For this review, use the dimensioned drawing (mm, ordinates from the lowest corner) and the shaded views. A direction names the side the tool comes from. Round coordinates to 2 decimals unless told otherwise and drop trailing zeros. Write each loop counter-clockwise with the first axis right and the second up, starting at its lowest first coordinate (ties: lowest second). Pieces come first, ordered by that corner, then holes. Notation, with made-up numbers: M -34,78.5 L 12,78.5 A29 ccw 12,100.5 Z; hole C 78.5,31.5 d8. An arc over 180 degrees is marked long. One line per question, with ' | ' between items. Start each with the question number.
Item 1: Add section D-D, the plane y = 50. State the section outline as (x, z) points.
Item 2: Add section A-A, the plane z = 9.5. State the section outline as (x, y) points, and give its area (3 significant figures).
Item 3: Machinability: for the marked faces 4 and 5, which of the approach directions +Z, -Z, +X, -X, +Y, -Y give a long, thin tool a straight path to every point of the face, cutting with its end or side? Answer none if there is none.
Item 4: Add section C-C, the plane x = 3. State the section outline as (y, z) points.
Item 5: For L1, parallel to X at y = 58, z = 16.75; L2, parallel to Z at x = 27, y = 31, list the stretches that pass through material, from the lowest coordinate up.
Item 6: Draft analysis for pull direction Y (two halves, no side actions). For the marked faces 1, 2 and 3, state which applies: released by +Y, released by -Y, zero draft, split by the parting line, or undercut.
Item 7: Add section B-B, the plane y = 65. State the section outline as (x, z) points, and give its area (3 significant figures).
Item 8: Insertion check: pin 1 Ø1 at (y, z) = (0.5, 9) entering from -X; pin 2 Ø1 at (x, y) = (7, 32) entering from +Z; pin 3 Ø5 at (x, z) = (31.5, 6.5) entering from +Y; pin 4 Ø5 at (y, z) = (32.5, 16.5) entering from +X. Each pin has a flat end and moves straight along its axis. Give the tip position at first contact, or say it passes through.
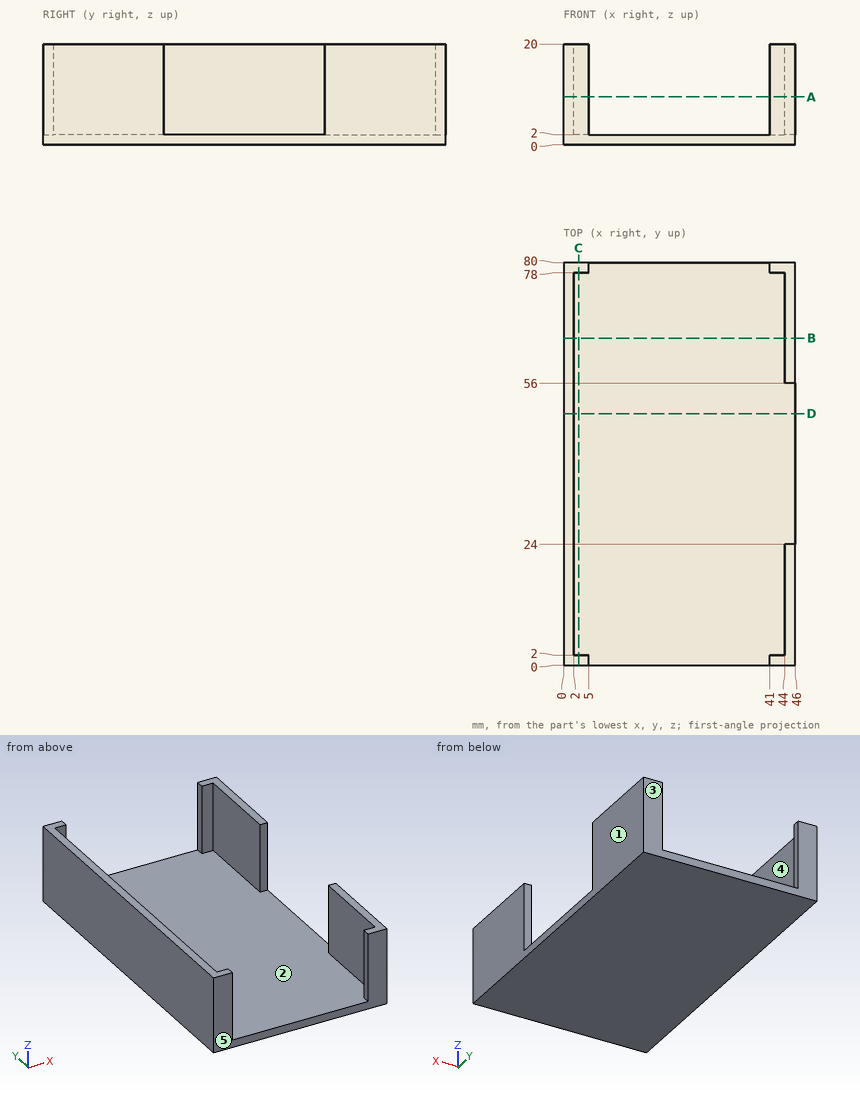
Computed values:
1) outline: M 0,0 L 46,0 L 46,2 L 2,2 L 2,20 L 0,20 Z
2) outline: M 0,0 L 5,0 L 5,2 L 2,2 L 2,78 L 5,78 L 5,80 L 0,80 Z; M 41,0 L 46,0 L 46,24 L 44,24 L 44,2 L 41,2 Z; M 41,78 L 44,78 L 44,56 L 46,56 L 46,80 L 41,80 Z | area: 280 mm^2
3) face 4: +Z | face 5: +Z, -Z, +X, -X, -Y
4) outline: M 0,0 L 80,0 L 80,20 L 78,20 L 78,2 L 2,2 L 2,20 L 0,20 Z
5) L1: x = 0 to 2, 44 to 46 | L2: z = 0 to 2
6) face 1: zero draft | face 2: undercut | face 3: released by +Y
7) outline: M 0,0 L 46,0 L 46,20 L 44,20 L 44,2 L 2,2 L 2,20 L 0,20 Z | area: 164 mm^2
8) pin 1: stops at x = 0 | pin 2: stops at z = 2 | pin 3: passes through | pin 4: stops at x = 2
